Autodesk Inventor part; units mm, degrees
ref_plane "YZ Plane" through (0, 0, 0) normal (1, 0, 0) x (0, 1, 0)
ref_plane "XZ Plane" through (0, 0, 0) normal (0, 1, 0) x (-1, 0, 0)
ref_plane "XY Plane" through (0, 0, 0) normal (0, 0, 1) x (1, 0, 0)
sketch "Sketch1" plane through (0, 0, 0) normal (0, 0, 1) x (1, 0, 0)
  line L0 (107.5, -20) -> (-107.5, -20)
  line L1 (-107.5, -20) -> (-107.5, 20)
  line L2 (-107.5, 20) -> (107.5, 20)
  line L3 (107.5, 20) -> (107.5, -20)
  line L4 (107.5, -20) -> (-107.5, 20) construction
  line L5 (-107.5, -20) -> (107.5, 20) construction
  arc A0 (-107.5, 20) -> (-107.5, -20) centre (-107.5, 0) ccw
  arc A1 (107.5, -20) -> (107.5, 20) centre (107.5, 0) ccw
  circle A2 centre (-107.5, 0) radius 3.5
  circle A3 centre (107.5, 0) radius 3.5
  point P0 (0, 0)
  dimension "d0" = 215
  dimension "d1" = 40
  dimension "d4" = 7
  dimension "d5" = 7
extrude "Extrusion1" add sketch "Sketch1" along normal blind 10 contours L0 L1 A2 L2 L3 A3 | L3 A3 A1 | A0 L1 A2
properties part number "Eslabon" material "Acetal Resin, White"
Could you check a few things on this model? Use its own coordinates, in mm. Round coordinates to 2 decimals unless told otherwise and drop trailing zeros. Write each loop counter-clockwise with the first axis right and the second up, starting at its lowest first coordinate (ties: lowest second). Pieces come first, ordered by that corner, then holes. Notation, with made-up numbers: (75, 6) - (79, 6) arc R15 ccw to (79, 34) - close; hole circle Ø3 at (53, -0.75). An arc over 180 degrees is marked (long way). Use a Markdown table: item, result.
Q1. I want a section at A-A (y = 0). List the corners of the cut face in (x, z) for me.
Output values:
| item | result |
|---|---|
| outline | (-127.5, 0) - (-111, 0) - (-111, 10) - (-127.5, 10) - close; (-104, 0) - (104, 0) - (104, 10) - (-104, 10) - close; (111, 0) - (127.5, 0) - (127.5, 10) - (111, 10) - close |
Q2. Please list where these lines run through material, in increasing order: L1, parallel to X at y = 0, z = 6.5; L2, parallel to Y at x = -107.5, z = 7.25; L3, parallel to X at y = 1.5, z = 3.75.
Output values:
| item | result |
|---|---|
| L1 | -127.5 to -111, -104 to 104, 111 to 127.5 |
| L2 | -20 to -3.5, 3.5 to 20 |
| L3 | -127.44 to -110.66, -104.34 to 104.34, 110.66 to 127.44 |
Q3. For pin 1 (4 mm diameter, centred on y = -10.5, z = 7.5, fed in from -X); pin 2 (5.5 mm diameter, centred on x = 107.5, y = 0, fed in from +Z); pin 3 (5 mm diameter, centred on y = 7.5, z = 1, fed in from +X), each with a flat end and sliding along its axis, tell me the tip position at first contact or that it passes through.
Output values:
| item | result |
|---|---|
| pin 1 | x = -125.6 |
| pin 2 | through |
| pin 3 | x = 126.86 |
Q4. Thinking about a two-plate mould opening in Y: for faces 1 (the cylindrical face through (127.495, 0.44, 4.93)), 2 (the flat face through (2, -20, 5)), 3 (the cylindrical face through (110.733, 1.341, 4.93)), which applies, released by +Y, released by -Y, zero draft, split by the parting line, or undercut?
Output values:
| item | result |
|---|---|
| face 1 | split by the parting line |
| face 2 | released by -Y |
| face 3 | undercut |
Q5. I want a section at C-C (y = -10). List the corners of the cut face in (x, z) for me.
Output values:
| item | result |
|---|---|
| outline | (-124.82, 0) - (124.82, 0) - (124.82, 10) - (-124.82, 10) - close |
Q6. I want a section at B-B (z = 2). List the corners of the cut face in (x, y) for me, plus the area to 3 significant figures.
Output values:
| item | result |
|---|---|
| outline | (-107.5, -20) - (107.5, -20) arc R20 ccw to (107.5, 20) - (-107.5, 20) arc R20 ccw to start; hole circle Ø7 at (-107.5, 0); hole circle Ø7 at (107.5, 0) |
| area | 9,780 mm2 |
